Input: dimensioned drawing with shaded views. Units: mm. Origin: part minimum x, y, z. A direction names the side the tool comes from. Round coordinates to 2 decimals unless told otherwise and drop trailing zeros. Loops run counter-clockwise (first coordinate to the right, second up) from the corner with the lowest first, then second, coordinate; pieces in that order, holes last. Notation, with made-up numbers: M -3,21 L 35,21 A27 ccw 35,48 Z; hole C 32,67 d8. An arc over 180 degrees is marked long. Write each question's results on one line, items separated by ' | '. Start each with the question number.
1. Draft query along Y for the marked faces 4 and 5. Return one class per face: released by +Y, released by -Y, zero draft, split by the parting line, or undercut.
2. Set-up query: the marked faces 1, 2 and 3. Return all of +Z, -Z, +X, -X, +Y, -Y with unobstructed straight access to the full face (end or side cutting, diameter ignored); none if empty.
3. Section B-B on z = 1. Output: boundary loops of the cut face in (x, y).
4. Contact query for flat-ended pins moving along their axis: pin 1 Ø1 at (y, z) = (7.5, 1.5) entering from -X; pin 2 Ø0.9 at (y, z) = (14, 1.5) entering from +X; pin 3 Ø0.9 at (y, z) = (13.5, 1) entering from -X. Output: stop coordinate, or through.
5. Ray query, line 1 (Y direction, x = 5, z = 1.6); line 2 (X direction, y = 5, z = 0.95); line 3 (Y direction, x = 5.5, z = 1.7). Return the intervals inside material, ascending.
6. Section C-C on x = 3.75. Output: boundary loops of the cut face in (y, z), and give its area (3 significant figures).
7. Section D-D on y = 8.5. Output: boundary loops of the cut face in (x, z).
8. Section A-A on x = 5. Output: boundary loops of the cut face in (y, z).
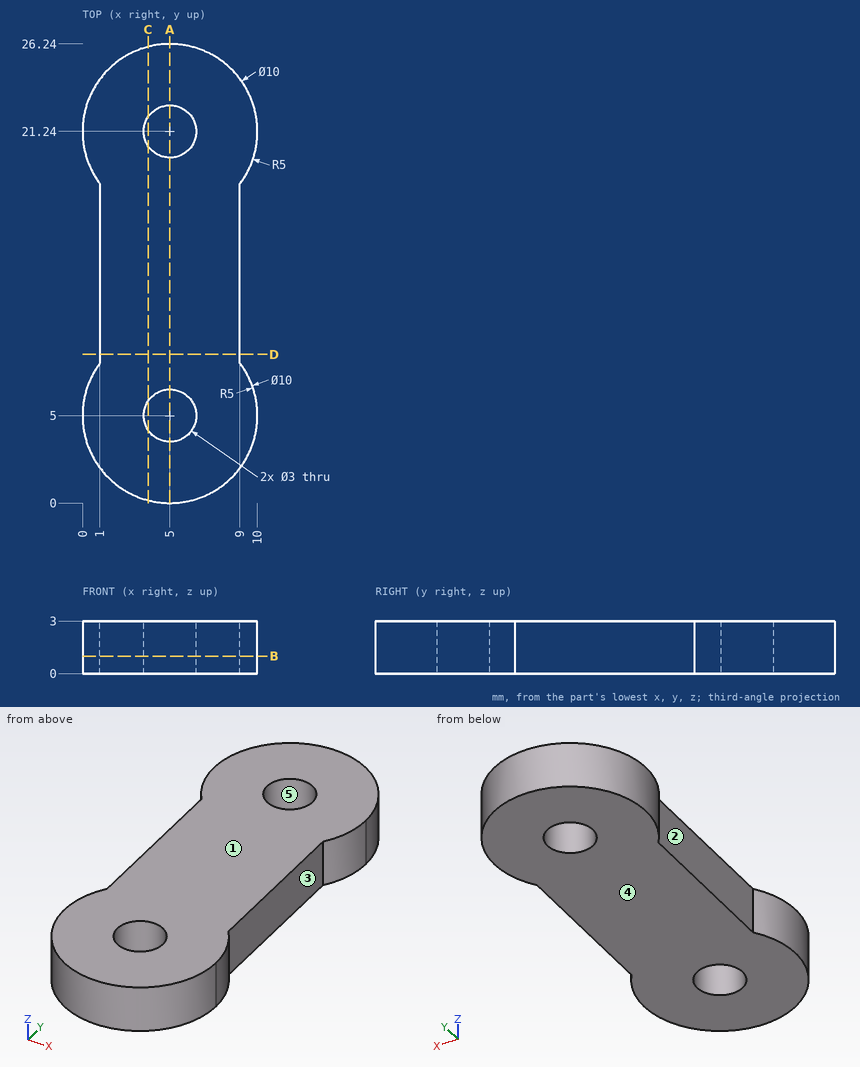
Taken from the geometry:
1) face 4: zero draft | face 5: undercut
2) face 1: +Z, +X, -X, +Y, -Y | face 2: +Z, -Z, -X | face 3: +Z, -Z, +X
3) outline: M 1,8 A5 ccw long 9,8 L 9,18.24 A5 ccw long 1,18.24 Z; hole C 5,5 d3; hole C 5,21.24 d3
4) pin 1: x = 0.42 | pin 2: x = 9 | pin 3: x = 1
5) line 1: 0 to 3.5, 6.5 to 19.74, 22.74 to 26.24 | line 2: 0 to 3.5, 6.5 to 10 | line 3: 0.03 to 3.59, 6.41 to 19.83, 22.65 to 26.21
6) outline: M 0.16,0 L 4.17,0 L 4.17,3 L 0.16,3 Z; M 5.83,0 L 20.41,0 L 20.41,3 L 5.83,3 Z; M 22.07,0 L 26.08,0 L 26.08,3 L 22.07,3 Z | area: 67.8 mm^2
7) outline: M 1,0 L 9,0 L 9,3 L 1,3 Z
8) outline: M 0,0 L 3.5,0 L 3.5,3 L 0,3 Z; M 6.5,0 L 19.74,0 L 19.74,3 L 6.5,3 Z; M 22.74,0 L 26.24,0 L 26.24,3 L 22.74,3 Z
